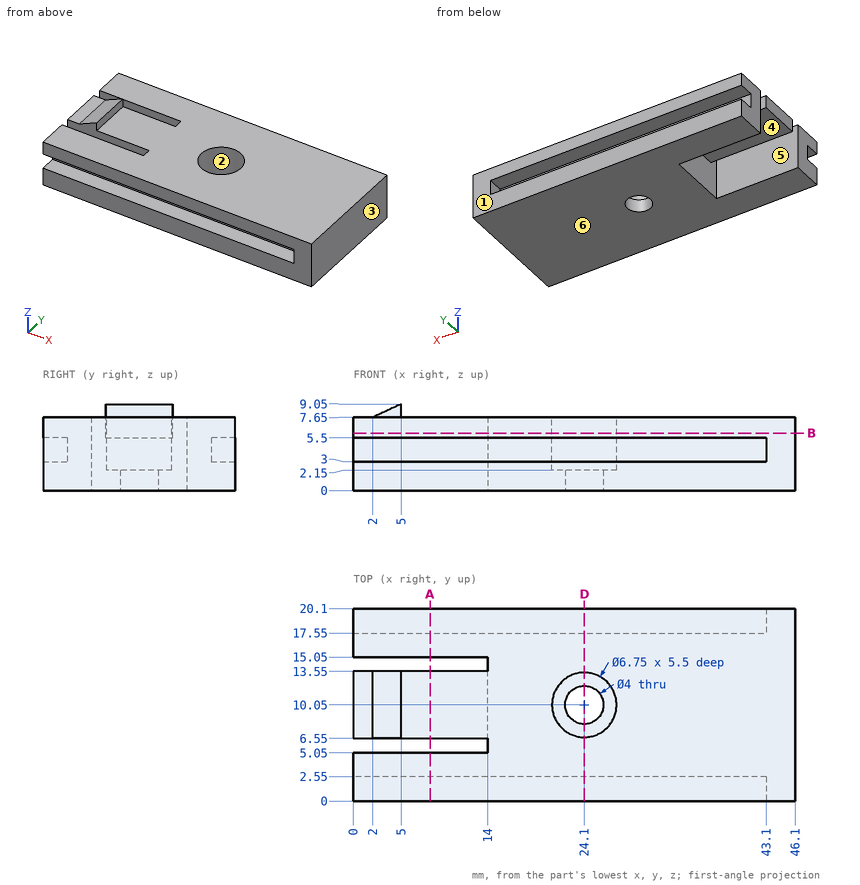
For this review, use the dimensioned drawing (mm, ordinates from the lowest corner) and the shaded views. A direction names the side the tool comes from. Coordinates: 2 decimals unless noted, no trailing zeros. Loops run counter-clockwise (first coordinate to the right, second up) from the corner with the lowest first, then second, coordinate; pieces in that order, holes last. Notation, with made-up numbers: (27.5, -24) -> (37.5, -24) arc R26 ccw to (37.5, 12) -> close; hole circle Ø5 at (12, 1). An arc over 180 degrees is marked (long way). Use a Markdown table: item, result. Add a question column.
Item 1: Clearance check with flat-ended pins moving along their axes: P1, Ø1.1, axis at y = 9.5, z = 8.5, coming from the +X side; P2, Ø4, axis at x = 14, y = 16.5, coming from the +Z side; P3, Ø1.2, axis at y = 0.5, z = 4.5, coming from the -X side. State where each tip first meets the part, or that it passes through.
Item 2: We need section A-A, the plane x = 8. Write out the cut boundary in (y, z), and give its area (3 significant figures).
Item 3: Wall thickness on L1, parallel to Y at x = 8, z = 6.5; L2, parallel to Y at x = 24.1, z = 1.25; L3, parallel to Y at x = 13, z = 2.25: over which ranges is each line inside the solid? List them lowest first. Write a range as from..to.
Item 4: We need section B-B, the plane z = 6. Write out the cut boundary in (x, y) (3 decimals).
Item 5: Machinability: for the marked faces 4, 5 and 6, which of the approach directions +Z, -Z, +X, -X, +Y, -Y give a long, thin tool a straight path to every point of the face, cutting with its end or side? Answer none if there is none.
Item 6: We need section D-D, the plane x = 24.1. Write out the cut boundary in (y, z) (3 decimals).
Item 7: The part is to be moulded in two halves that separate along Y. For the marked faces 1, 2 and 3, say which applies: +Y half, -Y half, draft (parallel to the pull), parting line (faces both ways), or undercut.
Numbers:
| question | item | result |
|---|---|---|
| 1 | P1 | stops at x = 5 |
| 1 | P2 | stops at z = 7.65 |
| 1 | P3 | stops at x = 43.1 |
| 2 | outline | (0, 0) -> (5.05, 0) -> (5.05, 7.65) -> (0, 7.65) -> (0, 5.5) -> (2.55, 5.5) -> (2.55, 3) -> (0, 3) -> close; (6.55, 5.5) -> (13.55, 5.5) -> (13.55, 7.65) -> (6.55, 7.65) -> close; (15.05, 0) -> (20.1, 0) -> (20.1, 3) -> (17.55, 3) -> (17.55, 5.5) -> (20.1, 5.5) -> (20.1, 7.65) -> (15.05, 7.65) -> close |
| 2 | area | 79.6 mm^2 |
| 3 | L1 | y = 0..5.05, 6.55..13.55, 15.05..20.1 |
| 3 | L2 | y = 0..8.05, 12.05..20.1 |
| 3 | L3 | y = 0..5.05, 15.05..20.1 |
| 4 | outline | (0, 0) -> (46.1, 0) -> (46.1, 20.1) -> (0, 20.1) -> (0, 15.05) -> (14, 15.05) -> (14, 13.55) -> (0, 13.55) -> (0, 6.55) -> (14, 6.55) -> (14, 5.05) -> (0, 5.05) -> close; hole circle Ø6.75 at (24.1, 10.05) |
| 5 | face 4 | -Z, -X |
| 5 | face 5 | +Z, -Z, -X |
| 5 | face 6 | -Z, +X, -X, +Y, -Y |
| 6 | outline | (0, 0) -> (8.05, 0) -> (8.05, 2.15) -> (6.675, 2.15) -> (6.675, 7.65) -> (0, 7.65) -> (0, 5.5) -> (2.55, 5.5) -> (2.55, 3) -> (0, 3) -> close; (12.05, 0) -> (20.1, 0) -> (20.1, 3) -> (17.55, 3) -> (17.55, 5.5) -> (20.1, 5.5) -> (20.1, 7.65) -> (13.425, 7.65) -> (13.425, 2.15) -> (12.05, 2.15) -> close |
| 7 | face 1 | +Y half |
| 7 | face 2 | undercut |
| 7 | face 3 | draft |
